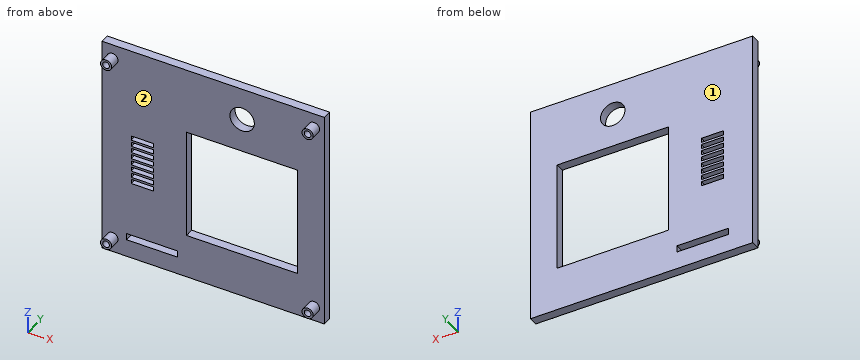
```python
from build123d import *

# Parameters (mm, degrees)
SKETCH2_W           = 100
SKETCH2_H           = 100
BOSS_EXTRUDE1_DEPTH = 4
SKETCH3_W           = 50
SKETCH3_H           = 50
CUT_EXTRUDE1_DEPTH  = 4
SKETCH4_W           = 23
SKETCH4_H           = 3
CUT_EXTRUDE2_DEPTH  = 4
SKETCH5_W           = 10
SKETCH5_H           = 2
CUT_EXTRUDE3_DEPTH  = 4
LPATTERN1_COUNT     = 8
LPATTERN1_PITCH     = 3
SKETCH6_R           = 5.5
CUT_EXTRUDE4_DEPTH  = 4
SKETCH8_R           = 2.5
BOSS_EXTRUDE3_DEPTH = 5
SKETCH10_R          = 1.5
CUT_EXTRUDE5_DEPTH  = 3
SKETCH11_R          = 1.5
CUT_EXTRUDE7_DEPTH  = 7
SKETCH12_R          = 1.5
CUT_EXTRUDE8_DEPTH  = 4
SKETCH13_R          = 1.5
CUT_EXTRUDE9_DEPTH  = 4
SKETCH14_R          = 1.5
CUT_EXTRUDE10_DEPTH = 4


with BuildPart() as part:
    # Sketch2 → Boss-Extrude1 (new body)
    with BuildSketch(Plane(origin=(0, 0, 0), x_dir=(1, 0, 0), z_dir=(0, 1, 0))):
        Rectangle(SKETCH2_W, SKETCH2_H)
    extrude(amount=BOSS_EXTRUDE1_DEPTH)

    # Sketch3 → Cut-Extrude1 (cut)
    with BuildSketch(Plane(origin=(0, 4, 0), x_dir=(1, 0, 0), z_dir=(0, 1, 0))):
        with Locations((13, 5)):
            Rectangle(SKETCH3_W, SKETCH3_H)
    extrude(amount=-CUT_EXTRUDE1_DEPTH, mode=Mode.SUBTRACT)

    # Sketch4 → Cut-Extrude2 (cut)
    with BuildSketch(Plane(origin=(0, 4, 0), x_dir=(1, 0, 0), z_dir=(0, 1, 0))):
        with Locations((-27.5, 40.5)):
            Rectangle(SKETCH4_W, SKETCH4_H)
    extrude(amount=-CUT_EXTRUDE2_DEPTH, mode=Mode.SUBTRACT)

    # Sketch5 → Cut-Extrude3 (cut)
    with BuildSketch(Plane(origin=(0, 4, 0), x_dir=(1, 0, 0), z_dir=(0, 1, 0))):
        with Locations((-31.87977559, 13)):
            Rectangle(SKETCH5_W, SKETCH5_H)
    cut_extrude3 = extrude(amount=-CUT_EXTRUDE3_DEPTH, mode=Mode.SUBTRACT)

    # LPattern1: Cut-Extrude3 ×8
    with Locations(*[(0, 0, i * LPATTERN1_PITCH) for i in range(1, LPATTERN1_COUNT)]):
        add(cut_extrude3, mode=Mode.SUBTRACT)

    # Sketch6 → Cut-Extrude4 (cut)
    with BuildSketch(Plane(origin=(0, 4, 0), x_dir=(1, 0, 0), z_dir=(0, 1, 0))):
        with Locations(Location((13, -35.361632217, 0), (0, 0, 270))):
            Circle(SKETCH6_R)
    extrude(amount=-CUT_EXTRUDE4_DEPTH, mode=Mode.SUBTRACT)

    # Sketch8 → Boss-Extrude3 (add)
    with BuildSketch(Plane(origin=(0, 0, 0), x_dir=(-1, 0, 0), z_dir=(0, -1, 0))):
        with Locations(Location((45.34, 43.34, 0), (0, 0, 270))):
            Circle(SKETCH8_R)
        with Locations(Location((-45.34, 43.34, 0), (0, 0, 270))):
            Circle(SKETCH8_R)
        with Locations(Location((-45.34, -43.34, 0), (0, 0, 270))):
            Circle(SKETCH8_R)
        with Locations(Location((45.339, -43.339, 0), (0, 0, 270))):
            Circle(SKETCH8_R)
    extrude(amount=BOSS_EXTRUDE3_DEPTH)

    # Sketch10 → Cut-Extrude5 (cut)
    with BuildSketch(Plane.XZ):
        with Locations(Location((-45.34, -43.34, 0), (0, 0, 270))):
            Circle(SKETCH10_R)
        with Locations(Location((45.318764469, -43.34, 0), (0, 0, 270))):
            Circle(SKETCH10_R)
    extrude(amount=-CUT_EXTRUDE5_DEPTH, mode=Mode.SUBTRACT)

    # Sketch11 → Cut-Extrude7 (cut)
    with BuildSketch(Plane.XZ):
        with Locations(Location((45.34, 43.34, 0), (0, 0, 270))):
            Circle(SKETCH11_R)
    extrude(amount=CUT_EXTRUDE7_DEPTH, mode=Mode.SUBTRACT)

    # Sketch12 → Cut-Extrude8 (cut)
    with BuildSketch(Plane.XZ.offset(5)):
        with Locations(Location((45.34, -43.34, 0), (0, 0, 270))):
            Circle(SKETCH12_R)
    extrude(amount=-CUT_EXTRUDE8_DEPTH, mode=Mode.SUBTRACT)

    # Sketch13 → Cut-Extrude9 (cut)
    with BuildSketch(Plane.XZ.offset(5)):
        with Locations(Location((-45.34, -43.34, 0), (0, 0, 270))):
            Circle(SKETCH13_R)
    extrude(amount=-CUT_EXTRUDE9_DEPTH, mode=Mode.SUBTRACT)

    # Sketch14 → Cut-Extrude10 (cut)
    with BuildSketch(Plane.XZ.offset(5)):
        with Locations(Location((-45.339, 43.339, 0), (0, 0, 270))):
            Circle(SKETCH14_R)
    extrude(amount=-CUT_EXTRUDE10_DEPTH, mode=Mode.SUBTRACT)


solid = part.part
```
The listing builds one solid part. Answer for the finished solid, in the listing's coordinates (mm). Face numbers are marked on the shaded views. Round coordinates to 2 decimals unless told otherwise and drop trailing zeros. Loops run counter-clockwise (first coordinate to the right, second up) from the corner with the lowest first, then second, coordinate; pieces in that order, holes last.
Q1. Find the intervals of material crossed by line 1 (X direction, y = -3.65, z = -43.34); line 2 (X direction, y = 2.25, z = -43.34); line 3 (Z direction, x = 28.5, y = 0.25), in increasing order.
Q2. Section B-B, the plane z = -18.5 is taken. Determine the outline of the cut face in (x, y), then the cut area to 3 significant figures.
Q3. For a pull along Z with two mould halves and no side action, classify the marked faces 1 and 2 as released by +Z, released by -Z, zero draft, split by the parting line, or undercut.
Q4. Section D-D, the plane z = -43.34 is taken. Determine the outline of the cut face in (x, y), then the cut area to 3 significant figures.
Q5. Section C-C, the plane x = -18.5 is taken. Determine the outline of the cut face in (y, z).
Q6. Given pin 1 Ø3 at (x, y) = (7.5, -2) entering from +Z; pin 2 Ø2.5 at (x, z) = (45.32, -43.34) entering from -Y, each flat-ended and moving along its own axis, determine where each tip first touches the part or whether it passes through.
Q7. Section A-A, the plane x = 13 is taken. Determine the outline of the cut face in (y, z).
Completed:
1. line 1: x = -47.84 to -46.84, -43.84 to -42.84, 42.84 to 43.84, 46.84 to 47.84
1. line 2: x = -50 to -46.84, -43.84 to 43.82, 46.82 to 50
1. line 3: z = -50 to -30, 20 to 50
2. outline: (-50, 0) - (-12, 0) - (-12, 4) - (-50, 4) - close; (38, 0) - (50, 0) - (50, 4) - (38, 4) - close
2. area: 200 mm2
3. face 1: zero draft
3. face 2: undercut
4. outline: (-50, 0) - (-47.84, 0) - (-47.84, -5) - (-46.84, -5) - (-46.84, -1) - (-43.84, -1) - (-43.84, -5) - (-42.84, -5) - (-42.84, 0) - (42.84, 0) - (42.84, -5) - (43.84, -5) - (43.84, -1) - (46.84, -1) - (46.84, -5) - (47.84, -5) - (47.84, 0) - (50, 0) - (50, 4) - (-50, 4) - close; hole (-46.84, 0) - (-43.84, 0) - (-43.84, 3) - (-46.84, 3) - close; hole (43.82, 0) - (46.82, 0) - (46.82, 3) - (43.82, 3) - close
4. area: 408 mm2
5. outline: (0, -50) - (4, -50) - (4, -42) - (0, -42) - close; (0, -39) - (4, -39) - (4, 50) - (0, 50) - close
6. pin 1: passes through
6. pin 2: stops at y = -1
7. outline: (0, -50) - (4, -50) - (4, -30) - (0, -30) - close; (0, 20) - (4, 20) - (4, 29.86) - (0, 29.86) - close; (0, 40.86) - (4, 40.86) - (4, 50) - (0, 50) - close
